from build123d import *

# Parameters (mm, degrees)
SKETCH1_R           = 2.667
BOSS_EXTRUDE1_DEPTH = 1.5875


with BuildPart() as part:
    # Sketch1 → Boss-Extrude1 (new body, symmetric)
    with BuildSketch(Plane(origin=(0, 0, 0), x_dir=(0, 0, -1), z_dir=(1, 0, 0))):
        with BuildLine():
            Line((-98.171, 17.907), (94.615, 17.907))
            Line((94.615, 17.907), (94.615, 13.462))
            Line((94.615, 13.462), (98.171, 13.462))
            Line((98.171, 13.462), (98.171, 4.826))
            Line((98.171, 4.826), (94.615, 4.826))
            Line((94.615, 4.826), (94.615, 2.667))
            Line((94.615, 2.667), (89.535, 2.667))
            Line((89.535, 2.667), (89.535, 4.191))
            Line((89.535, 4.191), (83.947, 4.191))
            Line((83.947, 4.191), (83.947, 2.667))
            Line((83.947, 2.667), (76.073, 2.667))
            Line((76.073, 2.667), (76.073, -2.667))
            Line((76.073, -2.667), (83.947, -2.667))
            Line((83.947, -2.667), (83.947, -4.191))
            Line((83.947, -4.191), (89.535, -4.191))
            Line((89.535, -4.191), (89.535, -2.667))
            Line((89.535, -2.667), (94.615, -2.667))
            Line((94.615, -2.667), (94.615, -4.826))
            Line((94.615, -4.826), (98.171, -4.826))
            Line((98.171, -4.826), (98.171, -13.462))
            Line((98.171, -13.462), (94.615, -13.462))
            Line((94.615, -13.462), (94.615, -17.907))
            Line((94.615, -17.907), (-98.171, -17.907))
            Line((-98.171, -17.907), (-98.171, -6.477))
            Line((-98.171, -6.477), (-80.391, -6.477))
            ThreePointArc((-80.391, -6.477), (-73.914, 0), (-80.391, 6.477))
            Line((-80.391, 6.477), (-98.171, 6.477))
            Line((-98.171, 6.477), (-98.171, 17.907))
        make_face()
        with Locations((-63.881, 10.287)):
            Circle(SKETCH1_R, mode=Mode.SUBTRACT)
        with Locations((-63.881, -10.287)):
            Circle(SKETCH1_R, mode=Mode.SUBTRACT)
        with Locations((-52.705, 0)):
            Circle(SKETCH1_R, mode=Mode.SUBTRACT)
        with Locations((-44.831, 11.303)):
            Circle(SKETCH1_R, mode=Mode.SUBTRACT)
        with Locations((21.717, 11.303)):
            Circle(SKETCH1_R, mode=Mode.SUBTRACT)
        with Locations((88.265, 11.303)):
            Circle(SKETCH1_R, mode=Mode.SUBTRACT)
        with Locations((88.265, -11.303)):
            Circle(SKETCH1_R, mode=Mode.SUBTRACT)
        with Locations((21.717, -11.303)):
            Circle(SKETCH1_R, mode=Mode.SUBTRACT)
        with Locations((-44.831, -11.303)):
            Circle(SKETCH1_R, mode=Mode.SUBTRACT)
        with Locations((-9.144, 10.795)):
            Circle(SKETCH1_R, mode=Mode.SUBTRACT)
        with Locations((-32.258, 10.795)):
            Circle(SKETCH1_R, mode=Mode.SUBTRACT)
        with Locations((66.802, 10.795)):
            Circle(SKETCH1_R, mode=Mode.SUBTRACT)
        with Locations((43.688, 10.795)):
            Circle(SKETCH1_R, mode=Mode.SUBTRACT)
        with Locations((43.688, -10.795)):
            Circle(SKETCH1_R, mode=Mode.SUBTRACT)
        with Locations((66.802, -10.795)):
            Circle(SKETCH1_R, mode=Mode.SUBTRACT)
        with Locations((-32.258, -10.795)):
            Circle(SKETCH1_R, mode=Mode.SUBTRACT)
        with Locations((-9.144, -10.795)):
            Circle(SKETCH1_R, mode=Mode.SUBTRACT)
        with Locations((-20.701, 0)):
            Circle(SKETCH1_R, mode=Mode.SUBTRACT)
        with Locations((55.245, 0)):
            Circle(SKETCH1_R, mode=Mode.SUBTRACT)
    extrude(amount=BOSS_EXTRUDE1_DEPTH, both=True)


solid = part.part
CAD build for the part. Positions are in the model's coordinates, mm. A direction names the side the tool comes from. Give positions to 0.01 mm unless a question says otherwise; leave off trailing zeros. Loops run counter-clockwise (first coordinate to the right, second up) from the corner with the lowest first, then second, coordinate; pieces in that order, holes last. Notation, with made-up numbers: M 45,-35 L 94,-35 A14 ccw 94,-8 Z; hole C -3.75,81 d5. An arc over 180 degrees is marked long. Answer in a Markdown table with one row per item. Add a question column.
Item 1: Band-saw the part on C-C on x = 0.3. Give the number of separate pieces and of enclosed holes in the cut face, then the cut area to 3 significant figures.
Item 2: Mould opens along Z. For faces 1 (the face through (0, 0, -76.073)), 2 (the face through (0, -12, 98.171)), 3 (the face through (-0.022, 9.172, -41.572)), 4 (the face through (0, 2.667, -92)) say: +Z half, -Z half, draft (parallel to the pull), parting line (faces both ways), or undercut.
Item 3: Drop flat-ended pins along their axis: P1, Ø6, axis at y = 11.303, z = -21.717, coming from the -X side; P2, Ø1.2, axis at x = 0, y = -3.5, coming from the +Z side. Give the stop position or say it passes through.
Item 4: Band-saw the part on B-B on z = 86.5. Give the cut face in (x, y), then the cut area to 3 significant figures.
Item 5: Tool access for faces 5 (the face through (0, -2.667, -92)), 6 (the face through (0, 6.477, 89)), 7 (the face through (-0.022, -10.678, -64.138)): list every direction of +Z, -Z, +X, -X, +Y, -Y with a clear straight run to the whole face (end or side of a thin tool).
Item 6: Probe probe 1 along Y at (x, z) = (1.15, 32); probe 2 along Z at (x, y) = (0.25, -2); probe 3 along Y at (x, z) = (1.4, -65). List the from-to ranges inside material, lowest first.
Item 7: Band-saw the part on A-A on y = 0. Give the cut face in (x, z).
Reply:
| question | item | result |
|---|---|---|
| 1 | separate pieces | 1 |
| 1 | enclosed holes | 19 |
| 1 | area | 6,130 mm^2 |
| 2 | face 1 | -Z half |
| 2 | face 2 | +Z half |
| 2 | face 3 | undercut |
| 2 | face 4 | draft |
| 3 | P1 | stops at x = -1.59 |
| 3 | P2 | stops at z = 75.38 |
| 4 | outline | M -1.59,-17.91 L 1.59,-17.91 L 1.59,-6.48 L -1.59,-6.48 Z; M -1.59,6.48 L 1.59,6.48 L 1.59,17.91 L -1.59,17.91 Z |
| 4 | area | 72.6 mm^2 |
| 5 | face 5 | -Z, +X, -X |
| 5 | face 6 | +Z, +X, -X |
| 5 | face 7 | +X, -X |
| 6 | probe 1 | y = -17.91 to -13.45, -8.14 to 8.14, 13.45 to 17.91 |
| 6 | probe 2 | z = -76.07 to -57.01, -53.48 to 18.94, 22.47 to 50.94, 54.47 to 74.23 |
| 6 | probe 3 | y = -17.91 to -12.76, -8.83 to 8.83, 12.76 to 17.91 |
| 7 | outline | M -1.59,-76.07 L 1.59,-76.07 L 1.59,-57.91 L -1.59,-57.91 Z; M -1.59,-52.58 L 1.59,-52.58 L 1.59,18.03 L -1.59,18.03 Z; M -1.59,23.37 L 1.59,23.37 L 1.59,50.04 L -1.59,50.04 Z; M -1.59,55.37 L 1.59,55.37 L 1.59,73.91 L -1.59,73.91 Z |
